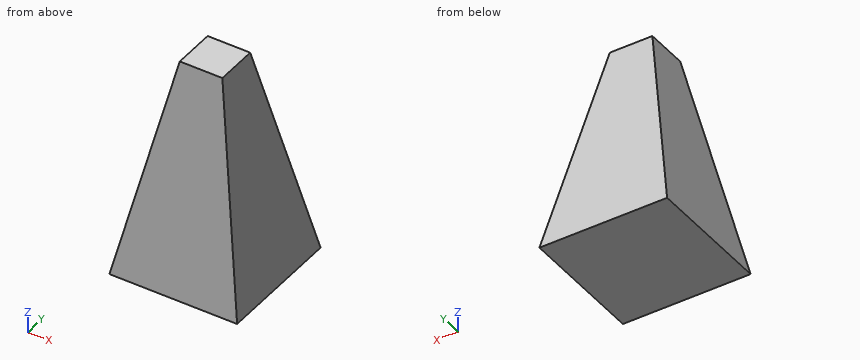
```python
from build123d import *

# Parameters (mm, degrees)
F0_W     = 76.2
F0_H     = 127
F1_DEPTH = 76.2
F3_DEPTH = 76.2
F5_DEPTH = 76.2


with BuildPart() as f1:
    # F0 (on Front) → F1 (new body)
    with BuildSketch(Plane.XZ):
        with Locations((38.1, 63.5)):
            Rectangle(F0_W, F0_H)
    extrude(amount=F1_DEPTH)

    # F2 (on face) → F3 (cut)
    with BuildSketch(Plane(origin=(0, 0, 0), x_dir=(0, -1, 0), z_dir=(-1, 0, 0))):
        Polygon((0, 127), (0, 0), (25.4, 127), align=None)
        Polygon((50.8, 127), (76.2, 0), (76.2, 127), align=None)
    extrude(amount=-F3_DEPTH, mode=Mode.SUBTRACT)

    # F4 (on Front) → F5 (cut)
    with BuildSketch(Plane.XZ):
        Polygon((0, 127), (0, 0), (25.4, 127), align=None)
        Polygon((50.8, 127), (76.2, 0), (76.2, 127), align=None)
    extrude(amount=F5_DEPTH, mode=Mode.SUBTRACT)


solid = f1.part
```
Part model, mm, in its own coordinate system. Round coordinates to 2 decimals unless told otherwise and drop trailing zeros. Loops run counter-clockwise (first coordinate to the right, second up) from the corner with the lowest first, then second, coordinate; pieces in that order, holes last. Notation, with made-up numbers: (-6.75, 60.5) -> (44.25, 60.5) arc R32 cw to (44.25, 94.5) -> close; hole circle Ø8 at (-4, -18.5). An arc over 180 degrees is marked (long way). Use one line per item in the form item = value. Start each with the question number.
Item 1: Drill centre lines: line 1 along X through (y, z) = (-55, 90); line 2 along X through (y, z) = (-22, 44); line 3 along Y through (x, z) = (34, 77.5). Where is each one in solid material? Low to high.
Item 2: Drop flat-ended pins along their axis: pin 1 Ø1.5 at (x, z) = (27.5, 81.5) entering from +Y; pin 2 Ø10 at (y, z) = (-66, 57) entering from -X; pin 3 Ø8 at (x, z) = (39, 114) entering from -Y; pin 4 Ø6 at (x, y) = (63, -18) entering from -Z. Give the stop position or say it passes through.
Item 3: Band-saw the part on A-A (z = 77.5). List the corners of the cut face in (x, y), plus the area to 3 significant figures.
Item 4: Band-saw the part on B-B (y = -66). List the corners of the cut face in (x, z).
Data:
q1.line_1 = 18 to 58.2
q1.line_2 = 8.8 to 67.4
q1.line_3 = -60.7 to -15.5
q2.pin_1 = -16.15
q2.pin_2 = 10.4
q2.pin_3 = -54.2
q2.pin_4 = 0
q3.outline = (15.5, -60.7) -> (60.7, -60.7) -> (60.7, -15.5) -> (15.5, -15.5) -> close
q3.area = 2,040 mm^2
q4.outline = (0, 0) -> (76.2, 0) -> (66, 51) -> (10.2, 51) -> close
